Part print with two shaded views. Sizes in mm from the minimum x, y, z corner. Give positions to 0.01 mm unless a question says otherwise; leave off trailing zeros. Write each loop counter-clockwise with the first axis right and the second up, starting at its lowest first coordinate (ties: lowest second). Pieces come first, ordered by that corner, then holes.
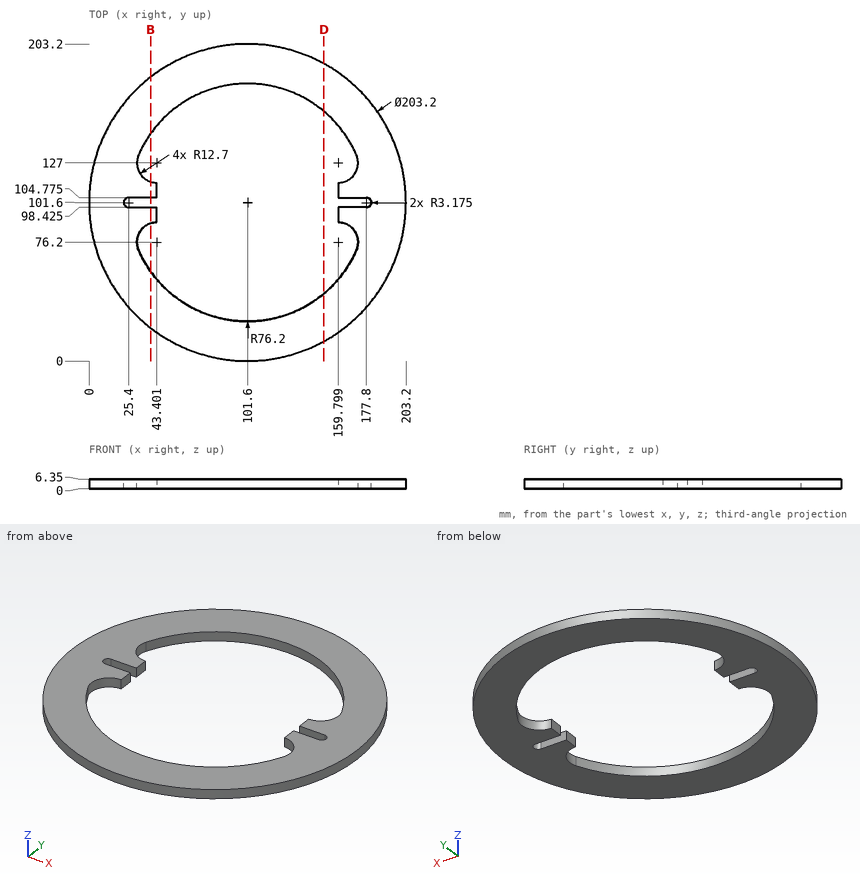
1) Saw through at B-B, the plane x = 39.5. Count the separate pieces of the cut face and the enclosed holes in it, then the cut area to 3 significant figures.
Answers follow:
separate pieces: 4
enclosed holes: 0
area: 589 mm2
2) Wall check: L1, parallel to Y at x = 39, z = 5.5 (1 decimal); L2, parallel to X at y = 42.5, z = 0.75; L3, parallel to X at y = 50.5, z = 3.75 (1 decimal). Give the ranges that are in metal, low to high.
Answers follow:
L1: y = 21.6 to 58.2, 88.1 to 98.4, 104.8 to 115.1, 145 to 181.6
L2: x = 18.96 to 53.5, 149.7 to 184.24
L3: x = 13.8 to 45.1, 158.1 to 189.4
3) Saw through at D-D, the plane x = 150.5. Write the cut outline in (y, z), then the cut area to 3 significant figures.
Answers follow:
outline: (12.54, 0) - (43.16, 0) - (43.16, 6.35) - (12.54, 6.35) - close; (160.04, 0) - (190.66, 0) - (190.66, 6.35) - (160.04, 6.35) - close
area: 389 mm2
4) Pin check, flat tips, straight feed: pin 1 Ø1.9 at (x, z) = (36.5, 2) entering from +Y; pin 2 Ø3 at (x, z) = (37.5, 4) entering from -Y; pin 3 Ø3 at (y, z) = (92.5, 4.5) entering from +X (1 decimal). Stop position of each tip, or through.
Answers follow:
pin 1: stops at y = 180.39
pin 2: stops at y = 21.58
pin 3: stops at x = 202.9
